Geometry: final body of the model. Coordinates: model frame, mm. Face numbers are marked on the shaded views. Give positions to 0.01 mm unless a question says otherwise; leave off trailing zeros. Write each loop counter-clockwise with the first axis right and the second up, starting at its lowest first coordinate (ties: lowest second). Pieces come first, ordered by that corner, then holes.
from build123d import *

# Parameters (mm, degrees)
BOSS_EXTRUDE1_DEPTH      = 17
BOSS_EXTRUDE1_DEPTH_BACK = 17
SKETCH4_R                = 1
CUT_EXTRUDE1_DEPTH       = 17


with BuildPart() as part:
    # Sketch1 → Boss-Extrude1 (new body, two sides)
    with BuildSketch(Plane(origin=(0, 0, 0), x_dir=(0, 0, -1), z_dir=(1, 0, 0))) as boss_extrude1_sk:
        with BuildLine():
            Line((0, 0), (1, 0))
            Line((1, 0), (1, 9))
            Line((1, 9), (-2.8, 9))
            Line((-2.8, 9), (-2.8, 0))
            Line((-2.8, 0), (-2.8, -4.689169104))
            Line((-2.8, -4.689169104), (-0.351186116, -8.93063917))
            Line((-0.351186116, -8.93063917), (0, -8.93063917))
            Line((0, -8.93063917), (0.3465, -8.93063917))
            add(Edge.make_bspline(
                [(0, -5.784861062), (0.068127357, -7.369329156), (0.3465, -8.93063917)],
                knots=[0, 0, 0, 1, 1, 1], degree=2))
            Line((0, -5.784861062), (0, 0))
        make_face()
    extrude(amount=BOSS_EXTRUDE1_DEPTH)
    extrude(boss_extrude1_sk.sketch, amount=-BOSS_EXTRUDE1_DEPTH_BACK)

    # Sketch4 → Cut-Extrude1 (cut)
    with BuildSketch(Plane(origin=(0, 0, -1), x_dir=(-1, 0, 0), z_dir=(0, 0, -1))):
        with Locations((-10, 3.95)):
            Circle(SKETCH4_R)
        with Locations((10, 3.95)):
            Circle(SKETCH4_R)
    extrude(amount=-CUT_EXTRUDE1_DEPTH, mode=Mode.SUBTRACT)


solid = part.part
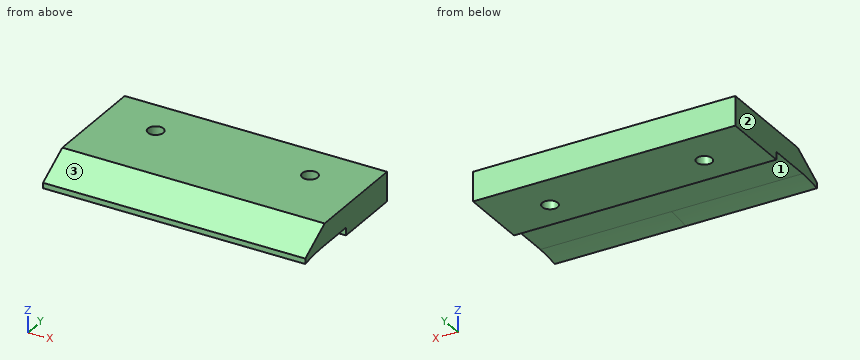
Q1. Section B-B on z = 1.35. Output: boundary loops of the cut face in (x, y).
Filled sheet:
outline: (-17, -7.2) - (17, -7.2) - (17, 9) - (-17, 9) - close; hole circle Ø2 at (-10, 3.95); hole circle Ø2 at (10, 3.95)
Q2. Pin query (flat end, axial travel): P1, Ø2.5, axis at x = -10, y = 3.95, coming from the +Z side; P2, Ø1, axis at x = 6.5, y = -6.5, coming from the +Z side; P3, Ø3, axis at x = 4, y = -4.5, coming from the -Z side. Return the tip coordinate at first contact, or that it passes through.
Filled sheet:
P1: stops at z = 2.8
P2: stops at z = 2.04
P3: stops at z = -0.01
Q3. Section A-A on y = 3.95. Output: boundary loops of the cut face in (x, z).
Filled sheet:
outline: (-17, -1) - (-11, -1) - (-11, 2.8) - (-17, 2.8) - close; (-9, -1) - (9, -1) - (9, 2.8) - (-9, 2.8) - close; (11, -1) - (17, -1) - (17, 2.8) - (11, 2.8) - close
Q4. Pull-direction query (Y, two-part tool) for the marked faces 1, 2 and 3; classes: released by +Y, released by -Y, zero draft, split by the parting line, or undercut.
Filled sheet:
face 1: undercut
face 2: zero draft
face 3: released by -Y
Q5. Ray query, line 1 along Z through (x, y) = (-7, -3.25); line 2 along Y through (x, z) = (-6, -0.4); line 3 along Y through (x, z) = (-10, 1.8). Return the intervals inside material, ascending.
Filled sheet:
line 1: z = 0 to 2.8
line 2: y = 0 to 9
line 3: y = -6.42 to 2.95, 4.95 to 9
Q6. Section C-C on y = -1.5. Output: boundary loops of the cut face in (x, z), plus the area to 3 significant figures.
Filled sheet:
outline: (-17, 0) - (17, 0) - (17, 2.8) - (-17, 2.8) - close
area: 95.2 mm2
